Geometry: final body of the model. Coordinates: model frame, mm. Face numbers are marked on the shaded views. Round coordinates to 2 decimals unless told otherwise and drop trailing zeros. Loops run counter-clockwise (first coordinate to the right, second up) from the corner with the lowest first, then second, coordinate; pieces in that order, holes last. Notation, with made-up numbers: (21, 76) - (51, 76) arc R10 ccw to (51, 86) - close; hole circle Ø10 at (-18, -8). An arc over 180 degrees is marked (long way). Write item = value, one per line. Start each with the question number.
Item 1: Section B-B (z = 3.8). Return loops of the section in (x, y).
Item 2: Section A-A (y = 2). Return loops of the section in (x, z), plus the area to 3 significant figures.
Item 3: Section D-D (x = -3). Return loops of the section in (y, z), plus the area to 3 significant figures.
Item 4: Draft query along Y for the marked faces 1, 2 and 3. Return one class per face: pulls with the +Y half, pulls with the -Y half, needs draft (parallel to the pull), parting line crosses it, or undercut.
Item 5: Section C-C (x = 2.5). Return loops of the section in (y, z), plus the area to 3 significant figures.
Item 6: Line query: line 1 (X direction, y = 2.75, z = 3.1); line 2 (Y direction, x = 2.5, z = 0.3); line 3 (Y direction, x = -1.75, z = 0.5). Output: solid intervals per line, ascending. Write a range as from..to.
Item 7: First-contact query: pin 1 (3 mm diameter, centred on x = -2, z = 1, fed in from +Y); pin 2 (2.5 mm diameter, centred on x = -2.5, y = 2, fed in from -Z). Flat tips, straight axial feed; report the tip coordinate or a pass-through.
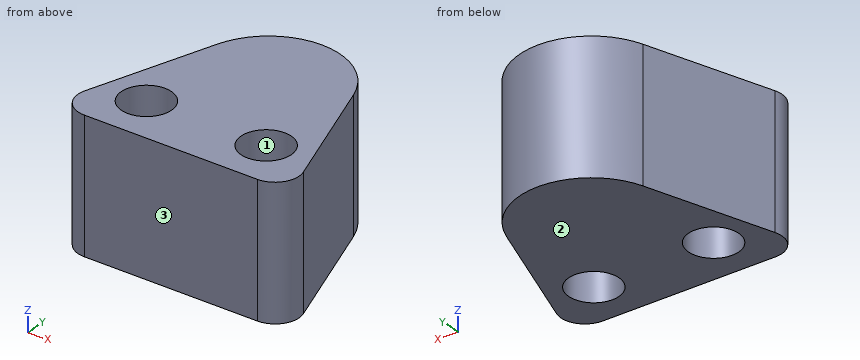
from build123d import *

# Parameters (mm, degrees)
EXTRUDE_1_DEPTH     = 5.5
FILLET_1_R          = 1
SKETCH_2_R          = 1.05
CUT_EXTRUDE_1_DEPTH = 17.629066118
FILLET_2_R          = 3


with BuildPart() as part:
    # ｽｹｯﾁ1 → ﾎﾞｽ - 押し出し1 (new body)
    with BuildSketch(Plane.XY):
        Polygon((-5, 0), (5, 0), (0, 15), align=None)
    extrude(amount=EXTRUDE_1_DEPTH)

    # ﾌｨﾚｯﾄ1
    fillet_1_edges = [part.edges().sort_by_distance(p)[0] for p in [
        (5, 0, 2.75),
        (-5, 0, 2.75),
    ]]
    fillet(fillet_1_edges, radius=FILLET_1_R)

    # ｽｹｯﾁ2 → ｶｯﾄ - 押し出し1 (cut, through all)
    with BuildSketch(Plane.XY.offset(5.5)):
        with Locations((-2.5, 2)):
            Circle(SKETCH_2_R)
        with Locations((2.5, 2)):
            Circle(SKETCH_2_R)
    extrude(amount=-CUT_EXTRUDE_1_DEPTH, mode=Mode.SUBTRACT)

    # ﾌｨﾚｯﾄ2
    fillet_2_edges = [part.edges().sort_by_distance(p)[0] for p in [
        (0, 15, 2.75),
    ]]
    fillet(fillet_2_edges, radius=FILLET_2_R)


solid = part.part
Taken from the geometry:
q1.outline = (-4.56, 1.32) arc R1 ccw to (-3.61, 0) - (3.61, 0) arc R1 ccw to (4.56, 1.32) - (2.85, 6.46) arc R3 ccw to (-2.85, 6.46) - close; hole circle Ø2.1 at (-2.5, 2); hole circle Ø2.1 at (2.5, 2)
q2.outline = (-4.33, 0) - (-3.55, 0) - (-3.55, 5.5) - (-4.33, 5.5) - close; (-1.45, 0) - (1.45, 0) - (1.45, 5.5) - (-1.45, 5.5) - close; (3.55, 0) - (4.33, 0) - (4.33, 5.5) - (3.55, 5.5) - close
q2.area = 24.6 mm^2
q3.outline = (0, 0) - (1.08, 0) - (1.08, 5.5) - (0, 5.5) - close; (2.92, 0) - (6, 0) - (6, 5.5) - (2.92, 5.5) - close
q3.area = 22.8 mm^2
q4.face_1 = undercut
q4.face_2 = needs draft
q4.face_3 = pulls with the -Y half
q5.outline = (0, 0) - (0.95, 0) - (0.95, 5.5) - (0, 5.5) - close; (3.05, 0) - (7.17, 0) - (7.17, 5.5) - (3.05, 5.5) - close
q5.area = 27.9 mm^2
q6.line_1 = -4.08..-3.23, -1.77..1.77, 3.23..4.08
q6.line_2 = 0..0.95, 3.05..7.17
q6.line_3 = 0..1.27, 2.73..7.95
q7.pin_1 = 8.47
q7.pin_2 = 0
